from build123d import *

# Parameters (mm, degrees)
F0_W     = 34.9
F0_H     = 1.1
F1_DEPTH = 110
F2_W     = 70
F2_H     = 1
F3_DEPTH = 1
F4_R     = 0.5


with BuildPart() as f1:
    # F0 (on Top) → F1 (new body)
    with BuildSketch(Plane.XY):
        Polygon((64.47826, 0), (-7.52174, 0), (-7.52174, -1), (27.37826, -1), (29.57826, -1), (64.47826, -1), align=None)
        with Locations((9.92826, -1.55)):
            Rectangle(F0_W, F0_H)
        with Locations((47.02826, -1.55)):
            Rectangle(F0_W, F0_H)
    extrude(amount=F1_DEPTH)

    # F2 (on face) → F3 (join)
    with BuildSketch(Plane(origin=(0, 0, 0), x_dir=(-1, 0, 0), z_dir=(0, 1, 0))):
        Polygon((7.52174, 0), (7.52174, 110), (6.52174, 110), (6.52174, 109), (6.52174, 1), (6.52174, 0), align=None)
        with Locations((-28.47826, 109.5)):
            Rectangle(F2_W, F2_H)
        Polygon((-63.47826, 109), (-63.47826, 110), (-64.47826, 110), (-64.47826, 0), (-63.47826, 0), (-63.47826, 1), align=None)
        with Locations((-28.47826, 0.5)):
            Rectangle(F2_W, F2_H)
    extrude(amount=F3_DEPTH)

    # F4
    f4_edges = [f1.edges().sort_by_distance(p)[0] for p in [
        (9.92826, -2.1, 110),
        (29.57826, -1.55, 110),
        (27.37826, -1.55, 110),
        (28.47826, -1, 110),
        (47.02826, -2.1, 110),
    ]]
    fillet(f4_edges, radius=F4_R)


solid = f1.part
Input: part model. Units: mm. Frame: model coordinates. Give positions to 0.01 mm unless a question says otherwise; leave off trailing zeros. Write each loop counter-clockwise with the first axis right and the second up, starting at its lowest first coordinate (ties: lowest second). Pieces come first, ordered by that corner, then holes.
Q1. First-contact query: P1, Ø0.8, axis at x = 31.5, y = 0.5, coming from the -Z side; P2, Ø2, axis at x = 32, z = 88, coming from the +Y side; P3, Ø0.7, axis at x = 28, z = 60.5, coming from the -Y side. Flat tips, straight axial feed; report the tip coordinate or a pass-through.
Q2. Section B-B, the plane z = 88. Output: boundary loops of the cut face in (x, y).
Q3. Material intervals for probe 1 along X at (y, z) = (-1.3, 70); probe 2 along Z at (x, y) = (47, 0.65); probe 3 along X at (y, z) = (0.5, 53.5), sorted ascending.
Q4. Section C-C, the plane y = 0.5. Output: boundary loops of the cut face in (x, z), plus the area to 3 significant figures.
Q5. Pull-direction query (X, two-part tool) for faces 1 (the face through (29, 0, 54)), 2 (the face through (-7.522, -1, 54)), 3 (the face through (28, -1, 54)), 4 (the face through (29, -0.6, 0)); classes: pulls with the +X half, pulls with the -X half, needs draft (parallel to the pull), parting line crosses it, or undercut.
Q6. Section A-A, the plane x = 38. Output: boundary loops of the cut face in (y, z).
Filled in:
1. P1: stops at z = 0
1. P2: stops at y = 0
1. P3: stops at y = -1
2. outline: (-7.52, -2.1) - (27.38, -2.1) - (27.38, -1) - (29.58, -1) - (29.58, -2.1) - (64.48, -2.1) - (64.48, 1) - (63.48, 1) - (63.48, 0) - (-6.52, 0) - (-6.52, 1) - (-7.52, 1) - close
3. probe 1: x = -7.52 to 27.38, 29.58 to 64.48
3. probe 2: z = 0 to 1, 109 to 110
3. probe 3: x = -7.52 to -6.52, 63.48 to 64.48
4. outline: (-7.52, 0) - (64.48, 0) - (64.48, 110) - (-7.52, 110) - close; hole (-6.52, 1) - (63.48, 1) - (63.48, 109) - (-6.52, 109) - close
4. area: 360 mm2
5. face 1: undercut
5. face 2: pulls with the -X half
5. face 3: undercut
5. face 4: needs draft
6. outline: (-2.1, 0) - (1, 0) - (1, 1) - (0, 1) - (0, 109) - (1, 109) - (1, 110) - (-1.6, 110) arc R0.5 ccw to (-2.1, 109.5) - close
